from build123d import *

# Parameters (mm, degrees)
SKETCH1_W                = 110
SKETCH1_H                = 190
BOSS_EXTRUDE1_DEPTH      = 6
M8_CLEARANCE_HOLE1_D     = 8.2
CUT_EXTRUDE1_REACH       = 111.936
SKETCH3_R                = 10
M8_CLEARANCE_HOLE2_D     = 8.2
M8_CLEARANCE_HOLE2_DEPTH = 19.75
M8_CLEARANCE_HOLE2_TIP   = 2.463528538


with BuildPart() as part:
    # Sketch1 → Boss-Extrude1 (new body)
    with BuildSketch(Plane.XY):
        Rectangle(SKETCH1_W, SKETCH1_H)
    extrude(amount=BOSS_EXTRUDE1_DEPTH)

    # M8 Clearance Hole1 (through all)
    with Locations(Plane(origin=(-50, 75, 6), x_dir=(1, 0, 0), z_dir=(0, 0, 1))):
        with Locations((0, 0), (100, 0), (100, -150), (0, -150)):
            Hole(M8_CLEARANCE_HOLE1_D / 2)

    # Sketch3 → Cut-Extrude1 (cut, up to next)
    with BuildSketch(Plane.XY.offset(6), mode=Mode.PRIVATE) as cut_extrude1_sk1:
        Circle(SKETCH3_R)
    cut_extrude1_tool1 = extrude(cut_extrude1_sk1.sketch, amount=-CUT_EXTRUDE1_REACH, mode=Mode.PRIVATE) & part.part
    add(cut_extrude1_tool1.solids().sort_by_distance((0, 0, 6))[0], mode=Mode.SUBTRACT)

    # M8 Clearance Hole2
    with Locations(Plane(origin=(-30, 20, 6), x_dir=(1, 0, 0), z_dir=(0, 0, 1))):
        with Locations((0, 0), (60, 0), (60, -40), (0, -40)):
            Hole(M8_CLEARANCE_HOLE2_D / 2, depth=M8_CLEARANCE_HOLE2_DEPTH)
            with Locations((0, 0, -(M8_CLEARANCE_HOLE2_DEPTH + M8_CLEARANCE_HOLE2_TIP / 2))):  # 118° drill point
                Cone(0, M8_CLEARANCE_HOLE2_D / 2, M8_CLEARANCE_HOLE2_TIP, mode=Mode.SUBTRACT)


solid = part.part
Verification items for the finished model (mm, model axes). Give positions to 0.01 mm unless a question says otherwise; leave off trailing zeros. Loops run counter-clockwise (first coordinate to the right, second up) from the corner with the lowest first, then second, coordinate; pieces in that order, holes last. Notation, with made-up numbers: (-24.5, -2.75) - (-10.5, -2.75) arc R28 cw to (-10.5, 31.25) - close; hole circle Ø10 at (-40, -21). An arc over 180 degrees is marked (long way). Write each question's results on one line, items separated by ' | '.
1) Sectioned sample at C-C on x = 30. Record the boundary of the cut face in (y, z), plus the area to 3 significant figures.
Solution:
outline: (-95, 0) - (-24.1, 0) - (-24.1, 6) - (-95, 6) - close; (-15.9, 0) - (15.9, 0) - (15.9, 6) - (-15.9, 6) - close; (24.1, 0) - (95, 0) - (95, 6) - (24.1, 6) - close | area: 1,040 mm2
2) Sectioned sample at D-D on z = 4.05. Count the separate pieces of the cut face and the enclosed holes in it, plus the area to 3 significant figures.
Solution:
separate pieces: 1 | enclosed holes: 9 | area: 20,200 mm2
3) Sectioned sample at A-A on x = 0. Record the boundary of the cut face in (y, z).
Solution:
outline: (-95, 0) - (-10, 0) - (-10, 6) - (-95, 6) - close; (10, 0) - (95, 0) - (95, 6) - (10, 6) - close
4) Sectioned sample at B-B on y = 20. Record the boundary of the cut face in (x, z).
Solution:
outline: (-55, 0) - (-34.1, 0) - (-34.1, 6) - (-55, 6) - close; (-25.9, 0) - (25.9, 0) - (25.9, 6) - (-25.9, 6) - close; (34.1, 0) - (55, 0) - (55, 6) - (34.1, 6) - close
5) Mould release check, pull along Y, two halves, no side actions. Record for faces 1 (the flat face through (55, -1, 3)), 2 (the flat face through (-1, 95, 3)), 3 (the cylindrical face through (-26.746, 17.505, 2.958)): pulls with the +Y half, pulls with the -Y half, needs draft (parallel to the pull), parting line crosses it, or undercut.
Solution:
face 1: needs draft | face 2: pulls with the +Y half | face 3: undercut
6) Material ranges on L1, parallel to Y at x = -30, z = 4.2; L2, parallel to Y at x = 50, z = 1.55; L3, parallel to X at y = -17, z = 5.3, recorded low to high. Write a range as from..to.
Solution:
L1: -95..-24.1, -15.9..15.9, 24.1..95 | L2: -95..-79.1, -70.9..70.9, 79.1..95 | L3: -55..-32.79, -27.21..27.21, 32.79..55
